```python
from build123d import *

# Parameters (mm, degrees)
SKETCH1_R                   = 13
BOSS_EXTRUDE1_DEPTH         = 20
BOSS_EXTRUDE2_DEPTH         = 82
FILLET1_RADIUS              = 32
FILLET1_LENGTH              = 20
SKETCH3_R                   = 25
SKETCH3_R_2                 = 13
BOSS_EXTRUDE3_DEPTH         = 3
CUT_EXTRUDE2_DEPTH          = 169.493417496
FILLET1_OF_MIRROR1_2_RADIUS = 32
FILLET1_OF_MIRROR1_2_LENGTH = 20
SKETCH5_R                   = 13
CUT_EXTRUDE3_DEPTH          = 169.493417496


with BuildPart() as part:
    # Sketch1 → Boss-Extrude1 (new body)
    with BuildSketch(Plane(origin=(0, 0, 0), x_dir=(1, 0, 0), z_dir=(0, 1, 0))):
        with BuildLine():
            Line((-68, 68), (-108, 68))
            Line((-108, 68), (-108, 8))
            ThreePointArc((-108, 8), (-98.627416998, -14.627416998), (-76, -24))
            Line((-76, -24), (-0.620811238, -24))
            Line((-0.620811238, -24), (76, -24))
            ThreePointArc((76, -24), (98.627416998, -14.627416998), (108, 8))
            Line((108, 8), (108, 68))
            Line((108, 68), (68, 68))
            Line((68, 68), (56.627416998, 56.627416998))
            Line((56.627416998, 56.627416998), (70.769552622, 42.485281374))
            Line((70.769552622, 42.485281374), (25.514718626, -2.769552622))
            Line((25.514718626, -2.769552622), (11.372583002, 11.372583002))
            Line((11.372583002, 11.372583002), (0, 0))
            Line((0, 0), (-11.372583002, 11.372583002))
            Line((-11.372583002, 11.372583002), (-25.514718626, -2.769552622))
            Line((-25.514718626, -2.769552622), (-70.769552622, 42.485281374))
            Line((-70.769552622, 42.485281374), (-56.627416998, 56.627416998))
            Line((-56.627416998, 56.627416998), (-68, 68))
        make_face()
        with Locations(Location((-76, 8, 0), (0, 0, 270))):
            Circle(SKETCH1_R, mode=Mode.SUBTRACT)
        with Locations(Location((76, 8, 0), (0, 0, 270))):
            Circle(SKETCH1_R, mode=Mode.SUBTRACT)
    extrude(amount=BOSS_EXTRUDE1_DEPTH)

    # Sketch1<3> → Boss-Extrude2 (add)
    with BuildSketch(Plane(origin=(0, 0, 0), x_dir=(1, 0, 0), z_dir=(0, 1, 0))):
        Polygon((-11.372583002, 11.372583002), (-56.627416998, 56.627416998), (-70.769552622, 42.485281374), (-25.514718626, -2.769552622), align=None)
    boss_extrude2 = extrude(amount=BOSS_EXTRUDE2_DEPTH)

    # Fillet1: full round fillet: the end face becomes a half cylinder, R = half its width
    fillet1_face = Plane((-41.071067812, 82, -26.928932188), x_dir=(0.707106781187, 0, -0.707106781187), z_dir=(0, 1, 0))  # on the end face: x along it, z out of the body
    fillet1_slab = fillet1_face.offset(-FILLET1_RADIUS / 2) * Box(FILLET1_LENGTH, 2 * FILLET1_RADIUS, FILLET1_RADIUS, mode=Mode.PRIVATE)  # the body's end, R deep
    fillet1_round = Plane((-41.071067812, 50, -26.928932188), x_dir=(0, 1, 0), z_dir=(0.707106781187, 0, -0.707106781187)) * Cylinder(FILLET1_RADIUS, FILLET1_LENGTH, mode=Mode.PRIVATE)  # its axis R under the face
    add(fillet1_slab - fillet1_round, mode=Mode.SUBTRACT)

    # Sketch3 → Boss-Extrude3 (add)
    with BuildSketch(Plane(origin=(-14.142135624, 0, 14.142135624), x_dir=(0.7071067811865487, 0, 0.7071067811865465), z_dir=(-0.7071067811865465, 0, 0.7071067811865487))):
        with Locations(Location((-48.083261121, 50, 0), (0, 0, 180))):
            Circle(SKETCH3_R)
        with Locations(Location((-47.165571339, 50, 0), (0, 0, 180))):
            Circle(SKETCH3_R_2, mode=Mode.SUBTRACT)
    boss_extrude3 = extrude(amount=BOSS_EXTRUDE3_DEPTH)

    # Sketch3<3> → Cut-Extrude2 (cut, through all)
    with BuildSketch(Plane(origin=(-14.142135624, 0, 14.142135624), x_dir=(0.7071067811865487, 0, 0.7071067811865465), z_dir=(-0.7071067811865465, 0, 0.7071067811865487))):
        with BuildLine():
            ThreePointArc((-60.165571339, 50), (-47.165571339, 37), (-34.165571339, 50))
            Line((-34.165571339, 50), (-60.165571339, 50))
        make_face()
        with BuildLine():
            Line((-60.165571339, 50), (-34.165571339, 50))
            ThreePointArc((-34.165571339, 50), (-47.165571339, 63), (-60.165571339, 50))
        make_face()
    extrude(amount=-CUT_EXTRUDE2_DEPTH, mode=Mode.SUBTRACT)

    # Mirror1: Boss-Extrude2, Boss-Extrude3 across plane
    add(boss_extrude2.mirror(Plane(origin=(0, 0, 0), x_dir=(0, 0, 1), z_dir=(1, 0, 0))))
    add(boss_extrude3.mirror(Plane(origin=(0, 0, 0), x_dir=(0, 0, 1), z_dir=(1, 0, 0))))

    # Fillet1 of Mirror1 2: full round fillet: the end face becomes a half cylinder, R = half its width
    fillet1_of_mirror1_2_face = Plane((41.071067812, 82, -26.928932188), x_dir=(-0.707106781187, 0, -0.707106781187), z_dir=(0, 1, 0))  # on the end face: x along it, z out of the body
    fillet1_of_mirror1_2_slab = fillet1_of_mirror1_2_face.offset(-FILLET1_OF_MIRROR1_2_RADIUS / 2) * Box(FILLET1_OF_MIRROR1_2_LENGTH, 2 * FILLET1_OF_MIRROR1_2_RADIUS, FILLET1_OF_MIRROR1_2_RADIUS, mode=Mode.PRIVATE)  # the body's end, R deep
    fillet1_of_mirror1_2_round = Plane((41.071067812, 50, -26.928932188), x_dir=(0, 1, 0), z_dir=(-0.707106781187, 0, -0.707106781187)) * Cylinder(FILLET1_OF_MIRROR1_2_RADIUS, FILLET1_OF_MIRROR1_2_LENGTH, mode=Mode.PRIVATE)  # its axis R under the face
    add(fillet1_of_mirror1_2_slab - fillet1_of_mirror1_2_round, mode=Mode.SUBTRACT)

    # Sketch5 → Cut-Extrude3 (cut, through all)
    with BuildSketch(Plane(origin=(14.142135624, 0, 14.142135624), x_dir=(0.7071067811865487, 0, -0.7071067811865465), z_dir=(0.7071067811865465, 0, 0.7071067811865487))):
        with Locations(Location((47.340345076, 49.832858071, 0), (0, 0, 46.811598371))):
            Circle(SKETCH5_R)
    extrude(amount=-CUT_EXTRUDE3_DEPTH, mode=Mode.SUBTRACT)


solid = part.part
```
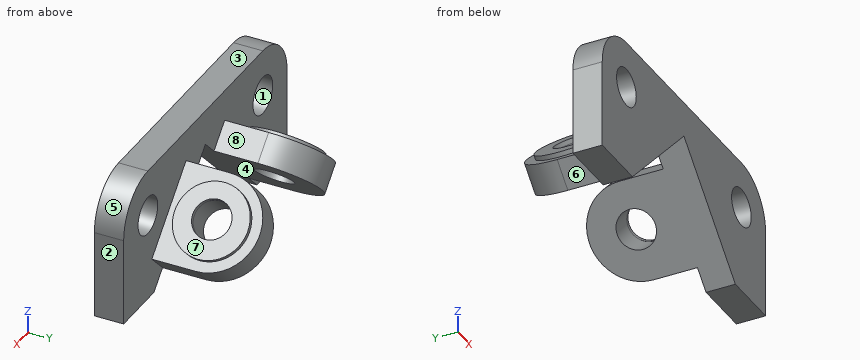
Could you check a few things on this model? Use its own coordinates, in mm. Face numbers are marked on the shaded views. A direction names the side the tool comes from. Give positions to 0.01 mm unless a question says otherwise; leave off trailing zeros. Order: outer loops, then holes, each group sorted by start corner. A loop starts at its lowest first (then second) coordinate and runs counter-clockwise, first axis right, second up.
Q1. If I drill on line 1 along X through (y, z) = (11.5, -8); line 2 along X through (y, z) = (5, -12); line 3 along Y through (x, z) = (97, -44.5), over which ranges is the centre line in solid material (lowest first)?
Q2. We'd pull the mould along Z, two halves only. Please class the marked faces 1, 2 and 3: +Z half, -Z half, draft (parallel to the pull), parting line (faces both ways), or undercut.
Q3. Suppose I cut it at A-A, the plane x = 81.5. Write out the boundary of the cut face in (y, z).
Q4. For the marked faces 4, 5, 6, 7 and 8, which set-ups out of +Z, -Z, +X, -X, +Y, -Y let a thin tool reach every point of the face, with its end or its side?
Q5. Suppose I cut it at C-C, the plane y = 13.5. Write out the boundary of the cut face in (x, z).
Q6. Suppose I cut it at D-D, the plane y = 57. Write out the boundary of the cut face in (x, z), and give its area (3 significant figures).
Q7. Suppose I cut it at B-B, the plane y = 48. Write out the boundary of the cut face in (x, z).
Q8. I'm going to push flat-ended pins straight in: P1, Ø8, axis at x = -56, y = 36.5, coming from the +Z side; P2, Ø12, axis at x = 25, y = 50.5, coming from the -Z side; P3, Ø2, axis at x = 51.5, y = 31.5, coming from the -Z side; P4, Ø8, axis at x = -48, z = 13.5, coming from the -Y side. Where does each tip first touch, or does it pass through?
Solution:
1. line 1: x = -108 to -89, -63 to -8, 8 to 63, 89 to 108
1. line 2: x = -108 to -88.37, -63.63 to -12, 12 to 63.63, 88.37 to 108
1. line 3: y = 0 to 20
2. face 1: undercut
2. face 2: draft
2. face 3: +Z half
3. outline: (0, -68) - (20, -68) - (20, -19.78) - (0, -19.78) - close; (0, 3.78) - (20, 3.78) - (20, 23.52) - (0, 23.52) - close
4. face 4: -Z, +Y, -Y
4. face 5: +Z, +X, +Y, -Y
4. face 6: -Z, -X, +Y
4. face 7: +Z, +X, +Y
4. face 8: +Z, +Y
5. outline: (-108, -68) - (-68, -68) - (0, 0) - (68, -68) - (108, -68) - (108, -8) arc R32 ccw to (76, 24) - (-76, 24) arc R32 ccw to (-108, -8) - close; hole circle Ø26 at (-76, -8); hole circle Ø26 at (76, -8)
6. outline: (-70.22, -41.94) - (-56.08, -56.08) - (-41.1, -41.1) - (-57.36, -24.83) - (-67.23, -34.71) - (-65.11, -36.83) - close; (-41.87, -9.34) - (-25.61, -25.61) - (-11.92, -11.92) - (-26.06, 2.22) - (-31.17, -2.89) - (-33.29, -0.77) - close; (11.92, -11.92) - (25.81, -25.81) - (39.95, -11.66) - (39.75, -11.46) - (41.87, -9.34) - (33.29, -0.77) - (31.17, -2.89) - (26.06, 2.22) - close; (41.14, -41.14) - (56.08, -56.08) - (70.22, -41.94) - (65.11, -36.83) - (67.23, -34.71) - (57.36, -24.83) - (55.24, -26.95) - (55.29, -27) - close
6. area: 1,780 mm2
7. outline: (-70.77, -42.49) - (-56.63, -56.63) - (-42.43, -42.43) - (-58.7, -26.17) - (-67.88, -35.36) - (-65.76, -37.48) - close; (-40.53, -8) - (-24.27, -24.27) - (-11.37, -11.37) - (-25.51, 2.77) - (-30.52, -2.24) - (-32.64, -0.12) - close; (11.37, -11.37) - (24.37, -24.37) - (38.52, -10.23) - (38.41, -10.13) - (40.53, -8) - (32.64, -0.12) - (30.52, -2.24) - (25.51, 2.77) - close; (42.58, -42.58) - (56.63, -56.63) - (70.77, -42.49) - (65.76, -37.48) - (67.88, -35.36) - (58.7, -26.17) - (56.58, -28.29) - (56.72, -28.43) - close
8. P1: stops at z = -19.47
8. P2: stops at z = -25.57
8. P3: stops at z = -52.5
8. P4: stops at y = 0
